from build123d import *

# Parameters (mm, degrees)
SKETCH_1_R               = 1
EXTRUDE_1_DEPTH          = 20
EXTRUDE_START            = -8.2
EXTRUDE_3_DEPTH          = 14
SKETCH_6_W               = 1.2
SKETCH_6_H               = 12
EXTRUDE_4_DEPTH          = 4
EXTRUDE_START_2          = -0.5
EXTRUDE_5_DEPTH          = 1.5
PATTERN_CIRCULAR_1_COUNT = 12
SKETCH_12_OUTSIDE_W      = 26.342
SKETCH_12_OUTSIDE_H      = 26.342
SKETCH_12_OUTSIDE_R      = 8
CUT_EXTRUDE_2_DEPTH      = 19.759656212


with BuildPart() as part:
    # 草图1 → 凸台-拉伸1 (new body)
    with BuildSketch(Plane(origin=(0, 0, 0), x_dir=(1, 0, 0), z_dir=(0, 1, 0))):
        with Locations(Location((0, 0, 0), (0, 0, 270))):
            Circle(SKETCH_1_R)
    extrude(amount=EXTRUDE_1_DEPTH)

    # 草图4 → 凸台-拉伸3 (add)
    with BuildSketch(Plane(origin=(0, 20, 0), x_dir=(1, 0, 0), z_dir=(0, 1, 0)).offset(EXTRUDE_START)):
        Polygon((4, 0), (3.464101615, 2), (2, 3.464101615), (0, 4), (-2, 3.464101615), (-3.464101615, 2), (-4, 0), (-3.464101615, -2), (-2, -3.464101615), (0, -4), (2, -3.464101615), (3.464101615, -2), align=None)
    extrude(amount=-EXTRUDE_3_DEPTH)

    # 草图6 → 凸台-拉伸4 (add)
    with BuildSketch(Plane(origin=(-3.732050808, 0, -1), x_dir=(-0.258819045102507, 0, 0.9659258262890721), z_dir=(-0.9659258262890721, 0, -0.258819045102507))):
        with Locations((0, 4.8)):
            Rectangle(SKETCH_6_W, SKETCH_6_H)
    extrude_4 = extrude(amount=EXTRUDE_4_DEPTH)

    # 草图7 → 凸台-拉伸5 (add)
    with BuildSketch(Plane(origin=(-7.595754113, 0, -2.03527618), x_dir=(-0.25881904510250703, 0, 0.9659258262890721), z_dir=(-0.9659258262890721, 0, -0.25881904510250703)).offset(EXTRUDE_START_2)):
        Polygon((1.03527618, 10.8), (-1.03527618, 10.8), (-1.03527618, -1.2), (1.03527618, -1), align=None)
    extrude_5 = extrude(amount=EXTRUDE_5_DEPTH)

    # 阵列(圆周)1: 凸台-拉伸4, 凸台-拉伸5 ×12 about axis
    pattern_circular_1_axis = Axis((0, 0, 0), (0, 1, 0))
    add([extrude_4.rotate(pattern_circular_1_axis, i * 360 / PATTERN_CIRCULAR_1_COUNT) for i in range(1, PATTERN_CIRCULAR_1_COUNT)])
    add([extrude_5.rotate(pattern_circular_1_axis, i * 360 / PATTERN_CIRCULAR_1_COUNT) for i in range(1, PATTERN_CIRCULAR_1_COUNT)])

    # 草图12 outside → 切除-拉伸2 (cut, through all)
    with BuildSketch(Plane(origin=(0, 11.8, 0), x_dir=(1, 0, 0), z_dir=(0, 1, 0))):
        Rectangle(SKETCH_12_OUTSIDE_W, SKETCH_12_OUTSIDE_H)
        Circle(SKETCH_12_OUTSIDE_R, mode=Mode.SUBTRACT)
    extrude(amount=-CUT_EXTRUDE_2_DEPTH, mode=Mode.SUBTRACT)


solid = part.part
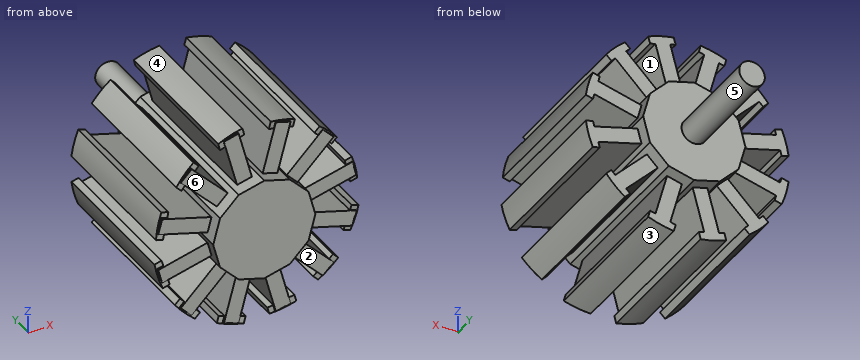
Model file for the job. Use its own axes, mm. Face numbers are marked on the shaded views. A direction names the side the tool comes from. Coordinates: 2 decimals unless noted, no trailing zeros. Order: outer loops, then holes, each group sorted by start corner. A loop starts at its lowest first (then second) coordinate and runs counter-clockwise, first axis right, second up. Notation, with made-up numbers: (62, 62.25) -> (112, 62.25) arc R17 cw to (112, 82.25) -> close; hole circle Ø8 at (43.5, 42.25). An arc over 180 degrees is marked (long way). Return JSON: item names as keys, results as strings. Group by question number.
Item 1: Tool access for the marked faces 4, 5 and 6: list every direction of +Z, -Z, +X, -X, +Y, -Y with a clear straight run to the whole face (end or side of a thin tool).
Item 2: Flat gauge pins, fed straight in: P1, Ø0.7, axis at x = -2, z = -6, coming from the -Y side; P2, Ø2, axis at x = -5, z = 4.5, coming from the +Y side; P3, Ø5, axis at x = 4.5, y = 8.5, coming from the -Z side. Where does each tip first touch, or does it go through?
Item 3: Pull direction X, two halves, no side cores. Call the marked faces 1, 2 and 3: pulls with the +X half, pulls with the -X half, needs draft (parallel to the pull), parting line crosses it, or undercut.
Item 4: Wall check: line 1 along Z through (x, y) = (5.75, 2.5); line 2 along X through (y, z) = (8.5, 5) (3 decimals); line 3 along X through (y, z) = (8.25, 6.25). Give the ranges that are in metal, low to high. Write a range as [from, to].
Item 5: Saw through at A-A on y = 18.75. Write the cut outline in (x, z).
Values found:
{
 "1": {"face 4": "+Z, -X, +Y, -Y", "face 5": "+Y", "face 6": "+Z, -X, -Y"},
 "2": {"P1": "stops at y = -1.2", "P2": "stops at y = 10.8", "P3": "stops at z = -7.75"},
 "3": {"face 1": "undercut", "face 2": "needs draft", "face 3": "pulls with the +X half"},
 "4": {"line 1": "z = [-5.56, -4.66], [-2.16, -0.92], [0.92, 2.16], [4.66, 5.56]", "line 2": "x = [-6.245, -4.151], [-1.961, -0.719], [0.719, 1.961], [4.151, 6.245]", "line 3": "x = [-4.99, -4.79], [-2.3, -1.05], [1.05, 2.3], [4.79, 4.99]"},
 "5": {"outline": "circle Ø2 at (0, 0)"}
}
